Can you work these out from the model? Positions are in its coordinate system, mm. A direction names the side the tool comes from. Give positions to 0.01 mm unless a question says otherwise; leave off trailing zeros. Write each loop counter-clockwise with the first axis right and the second up, starting at its lowest first coordinate (ties: lowest second). Pieces come first, ordered by that corner, then holes.
1. Suppose I cut it at B-B (x = 4.5). Please give me the cut outline in (y, z) (3 decimals), and give its area (3 significant figures).
2. Suppose I cut it at C-C (y = 0.9). Give the number of separate pieces and of enclosed holes in the cut face, and give its area (3 significant figures).
3. If I drill on probe 1 along Z at (x, y) = (0, 1.25); probe 2 along Z at (x, y) = (0, 2.75) (3 decimals); probe 3 along X at (y, z) = (0.65, 10), over which ranges is the centre line in solid material (lowest first)?
4. Suppose I cut it at A-A (z = 10). Please give me the cut outline in (x, y) (3 decimals).
5. On a 3-axis mill with a long thin cutter (end or side, diameter ignored), from which of +Z, -Z, +X, -X, +Y, -Y can I reach the whole of each face in a straight line? I mean faces 5 (the flat face through (1, 1.8, 1)), 6 (the cylindrical face through (-5.039, 1.479, -13.565)), 7 (the flat face through (-3.5, 1, 4)). Say none if no direction works.
6. I'm going to push flat-ended pins straight in: pin 1 (3 mm diameter, centred on x = 2, z = 9, fed in from -Y); pin 2 (0.9 mm diameter, centred on y = 1.5, z = 4, fed in from +X); pin 3 (2 mm diameter, centred on x = 0, z = 10, fed in from +Y); pin 4 (1.5 mm diameter, centred on y = 1.5, z = 0.5, fed in from -X). Where does each tip first touch, or does it pass through?
7. Suppose I cut it at D-D (z = 4.5). Please give me the cut outline in (x, y), and give its area (3 significant figures).
8. Thinking about a two-plate mould opening in Z: for faces 1 (the cylindrical face through (0.111, 0.887, -10.843)), 2 (the cylindrical face through (5.094, 1.479, -13.54)), 3 (the cylindrical face through (0.111, 0.887, 9.157)), 4 (the flat face through (3.5, 1, 4)), which applies, pulls with the +Z half, pulls with the -Z half, needs draft (parallel to the pull), parting line crosses it, or undercut?
```python
from build123d import *

# Parameters (mm, degrees)
BOSS_EXTRUDE1_DEPTH                          = 3
CBORE_FOR_M5_HEX_HEAD_BOLT1_D                = 1.7
CBORE_FOR_M5_HEX_HEAD_BOLT1_CBORE_D          = 3.25
CBORE_FOR_M5_HEX_HEAD_BOLT1_CBORE_DEPTH      = 1.2
FILLET1_R                                    = 5
FILLET2_R                                    = 3.5
FILLET3_R                                    = 3
CSK_FOR_M2_COUNTERSUNK_FLAT_HEAD_SCR_2_COUNT = 2
CSK_FOR_M2_COUNTERSUNK_FLAT_HEAD_SCR_2_PITCH = 9


with BuildPart() as part:
    # Sketch1 → Boss-Extrude1 (new body)
    with BuildSketch(Plane(origin=(0, 0, 0), x_dir=(1, 0, 0), z_dir=(0, 1, 0))):
        Polygon((3.5, 6), (8, 6), (8, 14), (-8, 14), (-8, 6), (-3.5, 6), (-3.5, -14), (3.5, -14), align=None)
    extrude(amount=BOSS_EXTRUDE1_DEPTH)

    # CBORE for M5 Hex Head Bolt1 (through all)
    with Locations(Plane(origin=(0, 3, 0), x_dir=(1, 0, 0), z_dir=(0, 1, 0))):
        with Locations((0, 10), (0, 0), (0, -10)):
            CounterBoreHole(CBORE_FOR_M5_HEX_HEAD_BOLT1_D / 2, CBORE_FOR_M5_HEX_HEAD_BOLT1_CBORE_D / 2, CBORE_FOR_M5_HEX_HEAD_BOLT1_CBORE_DEPTH)

    # Fillet1
    # the kernel refuses this fillet: 5 mm, written as the material it takes off along each edge
    with BuildSketch(Plane(origin=(-8, -12.437342964, -6), x_dir=(0, 0, -1), z_dir=(0, 1, 0))) as fillet1_piece_1:
        with BuildLine():
            CenterArc((4.974937186, -5), FILLET1_R, 90, 84.260829523)
            Line((0, -4.5), (-0.099498744, -4.49))
            ThreePointArc((-0.099498744, -4.49), (-0.1, -2.25), (-0.1, 0))
            Line((-0.1, 0), (0, 0.1))
            Line((0, 0.1), (4.974937186, 0.1))
            Line((4.974937186, 0.1), (4.974937186, 0))
        make_face()
    extrude(amount=27.874685928, mode=Mode.SUBTRACT)
    with BuildSketch(Plane(origin=(-8, -12.5, -14), x_dir=(1, 0, 0), z_dir=(0, 1, 0)), Plane(origin=(8, -12.5, -14), x_dir=(0, 0, 1), z_dir=(0, 1, 0))) as fillet1_piece_2:
        with BuildLine():
            CenterArc((FILLET1_R, -FILLET1_R), FILLET1_R, 90, 90)
            Line((0, -FILLET1_R), (-FILLET1_R * 0.02, -FILLET1_R))
            Line((-FILLET1_R * 0.02, -FILLET1_R), (-FILLET1_R * 0.02, FILLET1_R * 0.02))
            Line((-FILLET1_R * 0.02, FILLET1_R * 0.02), (FILLET1_R, FILLET1_R * 0.02))
            Line((FILLET1_R, FILLET1_R * 0.02), (FILLET1_R, 0))
        make_face()
    extrude(amount=28, mode=Mode.SUBTRACT)
    with BuildSketch(Plane(origin=(8, -12.437342964, -6), x_dir=(-1, 0, 0), z_dir=(0, 1, 0))) as fillet1_piece_3:
        with BuildLine():
            CenterArc((5, -4.974937186), FILLET1_R, 95.739170477, 84.260829523)
            Line((0, -4.974937186), (-0.1, -4.974937186))
            Line((-0.1, -4.974937186), (-0.1, 0))
            Line((-0.1, 0), (0, 0.1))
            ThreePointArc((0, 0.1), (2.25, 0.1), (4.49, 0.099498744))
            Line((4.49, 0.099498744), (4.5, 0))
        make_face()
    extrude(amount=27.874685928, mode=Mode.SUBTRACT)

    # Fillet2
    fillet2_edges = [part.edges().sort_by_distance(p)[0] for p in [
        (-7.901520762, 1.5, -9.987468593),
        (7.901520762, 1.5, -9.987468593),
    ]]
    fillet(fillet2_edges, radius=FILLET2_R)

    # Fillet3
    fillet3_edges = [part.edges().sort_by_distance(p)[0] for p in [
        (3.5, 1.5, -6),
        (3.5, 1.5, 14),
        (-3.5, 1.5, 14),
        (-3.5, 1.5, -6),
    ]]
    fillet(fillet3_edges, radius=FILLET3_R)

    # Sketch8 → CSK for M2 Countersunk Flat Head Screw2 (revolve, cut)
    with BuildSketch(Plane(origin=(-4.5, 0, -10), x_dir=(0, 0, -1), z_dir=(1, 0, 0))):
        Polygon((0, 0), (0, 3), (1.6, 3), (1.6, 3.375254051), (1.925, 0), align=None)
    csk_for_m2_countersunk_flat_head_screw2 = revolve(axis=Axis((-4.5, -6.35, -10), (0, 1, 0)), mode=Mode.SUBTRACT)

    # CSK for M2 Countersunk Flat Head Scr 2: CSK for M2 Countersunk Flat Head Screw2 ×2
    with Locations(*[(i * CSK_FOR_M2_COUNTERSUNK_FLAT_HEAD_SCR_2_PITCH, 0, 0) for i in range(1, CSK_FOR_M2_COUNTERSUNK_FLAT_HEAD_SCR_2_COUNT)]):
        add(csk_for_m2_countersunk_flat_head_screw2, mode=Mode.SUBTRACT)


solid = part.part
```
Checks:
1. outline: (0, -13.77) - (3, -13.77) - (3, -11.636) - (0, -11.925) - close; (0, -8.075) - (3, -8.364) - (3, -6.017) - (0, -6.017) - close
1. area: 12.6 mm2
2. separate pieces: 1
2. enclosed holes: 5
2. area: 216 mm2
3. probe 1: z = -14 to -10.85, -9.15 to -0.85, 0.85 to 9.15, 10.85 to 14
3. probe 2: z = -14 to -11.625, -8.375 to -1.625, 1.625 to 8.375, 11.625 to 14
3. probe 3: x = -3.5 to -0.85, 0.85 to 3.5
4. outline: (-3.5, 0) - (-0.85, 0) - (-0.85, 1.8) - (-1.625, 1.8) - (-1.625, 3) - (-3.5, 3) - close; (0.85, 0) - (3.5, 0) - (3.5, 3) - (1.625, 3) - (1.625, 1.8) - (0.85, 1.8) - close
5. face 5: +Y
5. face 6: -Z, -X, +Y, -Y
5. face 7: +Z, -X, +Y, -Y
6. pin 1: stops at y = 0
6. pin 2: stops at x = 3.5
6. pin 3: stops at y = 1.8
6. pin 4: stops at x = -3.5
7. outline: (-3.5, 0) - (3.5, 0) - (3.5, 3) - (-3.5, 3) - close
7. area: 21.0 mm2
8. face 1: undercut
8. face 2: pulls with the -Z half
8. face 3: undercut
8. face 4: needs draft
